from build123d import *

# Parameters (mm, degrees)
SKETCH1_R           = 31
SKETCH1_R_2         = 18
BOSS_EXTRUDE1_DEPTH = 5
SKETCH2_R           = 2.5
CUT_EXTRUDE1_DEPTH  = 83.445600309


with BuildPart() as part:
    # Sketch1 → Boss-Extrude1 (new body)
    with BuildSketch(Plane.XY):
        with Locations((-36.293764936, 16.369042749)):
            Circle(SKETCH1_R)
        with Locations((-36.275518266, 16.362982128)):
            Circle(SKETCH1_R_2, mode=Mode.SUBTRACT)
    extrude(amount=BOSS_EXTRUDE1_DEPTH)

    # Sketch2 → Cut-Extrude1 (cut, through all)
    with BuildSketch(Plane.XY.offset(5)):
        with Locations((-36.284641601, 40.866012439)):
            Circle(SKETCH2_R)
        with Locations((-15.059833215, 28.622398324)):
            Circle(SKETCH2_R)
        with Locations((-15.050709879, 4.119368013)):
            Circle(SKETCH2_R)
        with Locations((-36.26639493, -8.140048182)):
            Circle(SKETCH2_R)
        with Locations((-57.491203317, 4.103565933)):
            Circle(SKETCH2_R)
        with Locations((-57.500326652, 28.606596243)):
            Circle(SKETCH2_R)
    extrude(amount=-CUT_EXTRUDE1_DEPTH, mode=Mode.SUBTRACT)


solid = part.part
The model under review builds one solid part; all positions refer to its coordinate system, in mm. Round coordinates to 2 decimals unless told otherwise and drop trailing zeros. Order: outer loops, then holes, each group sorted by start corner. A loop starts at its lowest first (then second) coordinate and runs counter-clockwise, first axis right, second up. Notation, with made-up numbers: (47.25, 14) - (92.25, 14) arc R23 ccw to (92.25, 45) - close; hole circle Ø3 at (-13, 30.25). An arc over 180 degrees is marked (long way). Use one line per item in the form item = value.
Q1. Add section C-C on z = 4.25. Give the boundary of the cut face in (x, y), then the cut area to 3 significant figures.
Response values:
outline = circle Ø62 at (-36.29, 16.37); hole circle Ø5 at (-57.5, 28.61); hole circle Ø5 at (-57.49, 4.1); hole circle Ø36 at (-36.28, 16.36); hole circle Ø5 at (-36.28, 40.87); hole circle Ø5 at (-36.27, -8.14); hole circle Ø5 at (-15.06, 28.62); hole circle Ø5 at (-15.05, 4.12)
area = 1,880 mm^2
Q2. Add section A-A on x = -33. Give the boundary of the cut face in (y, z).
Response values:
outline = (-14.46, 0) - (-1.34, 0) - (-1.34, 5) - (-14.46, 5) - close; (34.06, 0) - (47.19, 0) - (47.19, 5) - (34.06, 5) - close
Q3. Clearance check with flat-ended pins moving along their axes: P1, Ø1.5, axis at y = 19, z = 4, coming from the +X side; P2, Ø2, axis at x = -12.5, z = 3, coming from the -Y side; P3, Ø1.5, axis at x = -18, z = 2.5, coming from the +Y side. State where each tip first meets the part, or that it passes through.
Response values:
P1 = -5.35
P2 = -4.64
P3 = 41.93
Q4. Add section D-D on y = -3. Give the boundary of the cut face in (x, z).
Response values:
outline = (-60.5, 0) - (-12.09, 0) - (-12.09, 5) - (-60.5, 5) - close
Q5. Mouldability with a two-part tool opening along X and no side actions: class faces 1 (the cylindrical face through (-19.63, 42.51, 2.46)), 2 (the flat face through (-23, 3, 0)), 3 (the cylindrical face through (-33.96, -9.1, 2.54)) as pulls with the +X half, pulls with the -X half, needs draft (parallel to the pull), parting line crosses it, or undercut.
Response values:
face_1 = parting line crosses it
face_2 = needs draft
face_3 = undercut
Q6. To check wall thickness, follow line 1 (X direction, y = 4, z = 2.2); line 2 (Y direction, x = -15, z = 3.65); line 3 (X direction, y = 30, z = 0.3). State the ranges of each line that lie inside material, in increasing order.
Response values:
line_1 = -64.72 to -59.99, -54.99 to -49.36, -23.19 to -17.55, -12.55 to -7.87
line_2 = -6.16 to 1.62, 6.62 to 26.12, 31.12 to 38.9
line_3 = -64.14 to -59.58, -55.42 to -48.02, -24.53 to -17.15, -12.97 to -8.45
Q7. Add section B-B on y = 25. Give the boundary of the cut face in (x, z), then the cut area to 3 significant figures.
Response values:
outline = (-66.07, 0) - (-52.07, 0) - (-52.07, 5) - (-66.07, 5) - close; (-20.48, 0) - (-6.52, 0) - (-6.52, 5) - (-20.48, 5) - close
area = 140 mm^2
